Could you check a few things on this model? Use its own coordinates, in mm. A direction names the side the tool comes from. Give positions to 0.01 mm unless a question says otherwise; leave off trailing zeros. Write each loop counter-clockwise with the first axis right and the second up, starting at its lowest first coordinate (ties: lowest second). Pieces come first, ordered by that corner, then holes. Notation, with made-up numbers: M 43.25,-31.5 L 91.25,-31.5 A27 cw 91.25,-9.5 Z; hole C 20,15 d9. An arc over 180 degrees is marked long. Use one line per item in the form item = value.
from build123d import *

# Parameters (mm, degrees)
Y_KSEKLIK_EKSTR_ZYON1_DEPTH      = 173
Y_KSEKLIK_EKSTR_ZYON1_DEPTH_BACK = 4.8
KES_EKSTR_ZYON3_DEPTH            = 196.216977169
KES_EKSTR_ZYON3_DEPTH_BACK       = 196.216977169
KES_EKSTR_ZYON6_DEPTH            = 196.216977169
KES_EKSTR_ZYON6_DEPTH_BACK       = 196.216977169
Y_KSEKLIK_EKSTR_ZYON3_DEPTH      = 3
Y_KSEKLIK_EKSTR_ZYON4_DEPTH      = 3
Y_KSEKLIK_EKSTR_ZYON5_DEPTH      = 3
IZIM12_W                         = 111.728887866
IZIM12_H                         = 42.234305359
Y_KSEKLIK_EKSTR_ZYON6_DEPTH      = 3
Y_KSEKLIK_EKSTR_ZYON7_DEPTH      = 3


with BuildPart() as part:
    # Çizim1 → Yükseklik-Ekstrüzyon1 (new, two sides: drawn at the far end of the back side and taken through both)
    with BuildSketch(Plane.XY.offset(-Y_KSEKLIK_EKSTR_ZYON1_DEPTH_BACK)):
        Polygon((52.033537584, 49.037416071), (-52.033537584, 49.037416071), (-76, 30.3), (-76, 0), (-73, 0), (-73, 28.837416071), (-51, 46.037416071), (51, 46.037416071), (73, 28.837416071), (73, 0), (76, 0), (76, 30.3), align=None)
    extrude(amount=Y_KSEKLIK_EKSTR_ZYON1_DEPTH + Y_KSEKLIK_EKSTR_ZYON1_DEPTH_BACK)

    # Çizim5 → Kes-Ekstrüzyon3 (cut, two sides: drawn at the far end of the back side and taken through both)
    with BuildSketch(Plane(origin=(0, 0, 0), x_dir=(0, 0, -1), z_dir=(1, 0, 0)).offset(-KES_EKSTR_ZYON3_DEPTH_BACK)):
        Polygon((-158, 49.037416071), (-173, 39.037416071), (-173, 49.037416071), align=None)
    extrude(amount=KES_EKSTR_ZYON3_DEPTH + KES_EKSTR_ZYON3_DEPTH_BACK, mode=Mode.SUBTRACT)

    # Çizim6 → Kes-Ekstrüzyon6 (cut, two sides: drawn at the far end of the back side and taken through both)
    with BuildSketch(Plane(origin=(0, 0, 0), x_dir=(1, 0, 0), z_dir=(0, 1, 0)).offset(-KES_EKSTR_ZYON6_DEPTH_BACK)):
        Polygon((76, -143), (76, -173), (52.033537584, -173), align=None)
        Polygon((-52.033537584, -173), (-76, -143), (-76, -173), align=None)
    extrude(amount=KES_EKSTR_ZYON6_DEPTH + KES_EKSTR_ZYON6_DEPTH_BACK, mode=Mode.SUBTRACT)

    # Çizim7 → Yükseklik-Ekstrüzyon3 (add)
    with BuildSketch(Plane(origin=(0, 106.87205728, 71.248038187), x_dir=(1, 0, 0), z_dir=(0, 0.8320502943378435, 0.5547001962252296))):
        Polygon((-55.864443933, -116.52736444), (55.864443933, -116.52736444), (58.220440286, -112.982967479), (52.033537584, -104.262882189), (-52.033537584, -104.262882189), (-58.220440286, -112.982967479), align=None)
    extrude(amount=-Y_KSEKLIK_EKSTR_ZYON3_DEPTH)

    # Çizim9 → Yükseklik-Ekstrüzyon4 (add)
    with BuildSketch(Plane(origin=(-116.126649253, 0, 92.771499161), x_dir=(0.6241623263226247, 0, 0.7812946885775748), z_dir=(-0.7812946885775748, 0, 0.6241623263226247))):
        Polygon((92.774277659, 44.200383049), (96.548930908, 42.234305359), (96.548930908, 0), (64.288803666, 0), (64.288803666, 30.3), align=None)
    extrude(amount=-Y_KSEKLIK_EKSTR_ZYON4_DEPTH)

    # Çizim10 → Yükseklik-Ekstrüzyon5 (add)
    with BuildSketch(Plane(origin=(116.126649253, 0, 92.771499161), x_dir=(0.6241623263226247, 0, -0.7812946885775748), z_dir=(0.7812946885775748, 0, 0.6241623263226247))):
        Polygon((-96.548930908, 42.234305359), (-96.548930908, 0), (-64.288803666, 0), (-64.288803666, 30.3), (-92.774277659, 44.200383049), align=None)
    extrude(amount=-Y_KSEKLIK_EKSTR_ZYON5_DEPTH)

    # Çizim12 → Yükseklik-Ekstrüzyon6 (add)
    with BuildSketch(Plane(origin=(0, 0, 168.2), x_dir=(-1, 0, 0), z_dir=(0, 0, -1))):
        with Locations((0, 21.11715268)):
            Rectangle(IZIM12_W, IZIM12_H)
    extrude(amount=Y_KSEKLIK_EKSTR_ZYON6_DEPTH)

    # Çizim13 → Yükseklik-Ekstrüzyon7 (add)
    with BuildSketch(Plane(origin=(0, 0, -4.8), x_dir=(-1, 0, 0), z_dir=(0, 0, -1))):
        Polygon((-76, 30.3), (-52.033537584, 49.037416071), (52.033537584, 49.037416071), (76, 30.3), (76, 0), (42.425, 0), (42.425, -10), (-42.425, -10), (-42.425, 0), (-76, 0), align=None)
    extrude(amount=Y_KSEKLIK_EKSTR_ZYON7_DEPTH)


solid = part.part
1) If I drill on L1, parallel to X at y = 20.5, z = 48; L2, parallel to Z at x = 4.5, y = 35.5; L3, parallel to Y at x = -3, z = 3.5, over which ranges is the centre line in solid material (lowest first)?
Checked values:
L1 = -76 to -73, 73 to 76
L2 = -7.8 to -4.8, 165.2 to 168.2
L3 = 46.04 to 49.04
2) For faces 1 (the flat face through (-0.815, 45.683, 163.031)), 2 (the flat face through (-0.79, 43.37, 161.09)), which set-ups out of +Z, -Z, +X, -X, +Y, -Y let a thin tool reach every point of the face, with its end or its side?
Checked values:
face_1 = +Z, +X, -X, +Y
face_2 = -Y
3) I want a section at C-C, the plane z = 65.5. Please give me the cut outline in (x, y).
Checked values:
outline = M -76,0 L -73,0 L -73,28.84 L -51,46.04 L 51,46.04 L 73,28.84 L 73,0 L 76,0 L 76,30.3 L 52.03,49.04 L -52.03,49.04 L -76,30.3 Z
4) Thinking about a two-plate mould opening in X: for faces 3 (the flat face through (76, 15, 69)), 4 (the flat face through (-63.58, 16.64, 153.74)), 5 (the flat face through (1, 49.037, 76)), 6 (the flat face through (73, 15, 68)), which applies, released by +X, released by -X, zero draft, split by the parting line, or undercut?
Checked values:
face_3 = released by +X
face_4 = undercut
face_5 = zero draft
face_6 = undercut
5) For pin 1 Ø3 at (x, z) = (17, 112.5) entering from -Y; pin 2 Ø21 at (x, y) = (-8, 11) entering from +Z; pin 3 Ø2.5 at (y, z) = (-7.5, -5.5) entering from +X (3 decimals), each with a flat end and sliding along its axis, tell me the tip position at first contact or that it passes through.
Checked values:
pin_1 = 46.04
pin_2 = 168.2
pin_3 = 42.425
6) I want a section at D-D, the plane x = 61. Please give me the cut outline in (y, z).
Checked values:
outline = M 0,-7.8 L 42.03,-7.8 L 42.03,161.78 L 0,161.78 L 0,156.97 L 38.22,156.97 L 38.22,-4.8 L 0,-4.8 Z
